```python
from build123d import *

# Parameters (mm, degrees)
SCHIZZO1_R                   = 4
SCHIZZO1_R_2                 = 10.5
SCHIZZO1_R_3                 = 3
ESTRUSIONE_ESTRUSIONE2_DEPTH = 10
SCHIZZO2_R                   = 2
TAGLIO_ESTRUSIONE1_DEPTH     = 15


with BuildPart() as part:
    # Schizzo1 → Estrusione-Estrusione2 (new body)
    with BuildSketch(Plane.XY):
        with BuildLine():
            Line((20, 0), (87.022408988, 0))
            ThreePointArc((87.022408988, 0), (97.768401155, 3.132171084), (105.148564729, 11.547634765))
            Line((105.148564729, 11.547634765), (242.445343973, 305.981528018))
            ThreePointArc((242.445343973, 305.981528018), (243.845108375, 310.105100974), (244.319188233, 314.433893253))
            Line((244.319188233, 314.433893253), (244.319188233, 380))
            ThreePointArc((244.319188233, 380), (238.461323856, 394.142135624), (224.319188233, 400))
            Line((224.319188233, 400), (166.622932407, 400))
            ThreePointArc((166.622932407, 400), (155.87694024, 396.867828916), (148.496776667, 388.452365235))
            Line((148.496776667, 388.452365235), (1.873844259, 74.018471982))
            ThreePointArc((1.873844259, 74.018471982), (0.474079858, 69.894899026), (0, 65.566106747))
            Line((0, 65.566106747), (0, 20))
            ThreePointArc((0, 20), (5.857864376, 5.857864376), (20, 0))
        make_face()
        with Locations((39.213445393, 53)):
            Circle(SCHIZZO1_R, mode=Mode.SUBTRACT)
        with Locations(Location((65.213445393, 53, 0), (0, 0, 180))):
            Circle(SCHIZZO1_R, mode=Mode.SUBTRACT)
        with Locations((65.213445393, 27)):
            Circle(SCHIZZO1_R, mode=Mode.SUBTRACT)
        with Locations(Location((39.213445393, 27, 0), (0, 0, 180))):
            Circle(SCHIZZO1_R, mode=Mode.SUBTRACT)
        with Locations((199.319188233, 355.469283566)):
            Circle(SCHIZZO1_R_2, mode=Mode.SUBTRACT)
        with Locations((183.819188233, 383.469283566)):
            Circle(SCHIZZO1_R_3, mode=Mode.SUBTRACT)
        with Locations((214.819188233, 383.469283566)):
            Circle(SCHIZZO1_R_3, mode=Mode.SUBTRACT)
        with Locations((220.532391668, 376.682487002)):
            Circle(SCHIZZO1_R_3, mode=Mode.SUBTRACT)
        with Locations((220.532391668, 334.256080131)):
            Circle(SCHIZZO1_R_3, mode=Mode.SUBTRACT)
        with Locations((214.819188233, 327.469283566)):
            Circle(SCHIZZO1_R_3, mode=Mode.SUBTRACT)
        with Locations((183.819188233, 327.469283566)):
            Circle(SCHIZZO1_R_3, mode=Mode.SUBTRACT)
        with Locations((178.105984797, 334.256080131)):
            Circle(SCHIZZO1_R_3, mode=Mode.SUBTRACT)
        with Locations((178.105984797, 376.682487002)):
            Circle(SCHIZZO1_R_3, mode=Mode.SUBTRACT)
    extrude(amount=-ESTRUSIONE_ESTRUSIONE2_DEPTH)

    # Schizzo2 → Taglio-Estrusione1 (cut)
    with BuildSketch(Plane.XZ):
        with Locations((53.511204494, -5)):
            Circle(SCHIZZO2_R)
        with Locations((81.011204494, -5)):
            Circle(SCHIZZO2_R)
        with Locations(Location((26.011204494, -5, 0), (0, 0, 180))):
            Circle(SCHIZZO2_R)
    extrude(amount=-TAGLIO_ESTRUSIONE1_DEPTH, mode=Mode.SUBTRACT)


solid = part.part
```
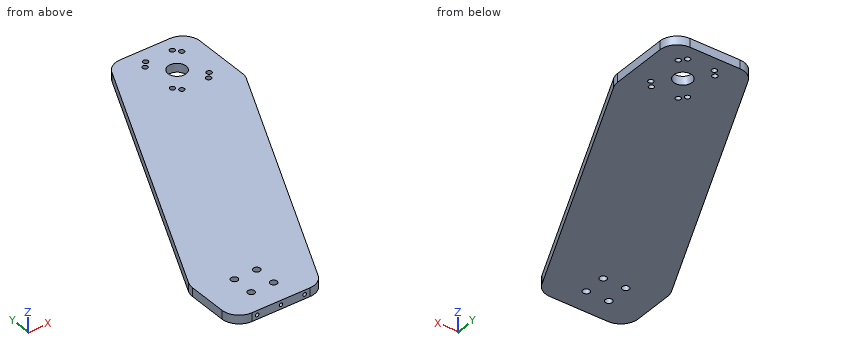
Geometry: final body of the model. Coordinates: model frame, mm. Coordinates: 2 decimals unless noted, no trailing zeros. Order: outer loops, then holes, each group sorted by start corner. A loop starts at its lowest first (then second) coordinate and runs counter-clockwise, first axis right, second up. Notation, with made-up numbers: (28.5, 85.25) - (39.5, 85.25) arc R31 ccw to (39.5, 119.25) - close; hole circle Ø3 at (11, 45.25). An arc over 180 degrees is marked (long way). Write each question's results on one line, items separated by ' | '.
(1) First-contact query: pin 1 Ø4 at (x, z) = (102.5, -8) entering from -Y; pin 2 Ø2.5 at (x, z) = (81.01, -5) entering from +Y; pin 3 Ø5 at (y, z) = (137.5, -1.5) entering from +X. Flat tips, straight axial feed; report the tip coordinate or a pass-through.
Values found:
pin 1: stops at y = 5.22 | pin 2: stops at y = 246.41 | pin 3: stops at x = 165.05
(2) Section query A-A, the plane y = 53. Return the cut outline in (x, z).
Values found:
outline: (0, -10) - (35.21, -10) - (35.21, 0) - (0, 0) - close; (43.21, -10) - (61.21, -10) - (61.21, 0) - (43.21, 0) - close; (69.21, -10) - (124.48, -10) - (124.48, 0) - (69.21, 0) - close
(3) Section query D-D, the plane y = 183. Return the cut outline in (x, z).
Values found:
outline: (52.69, -10) - (185.1, -10) - (185.1, 0) - (52.69, 0) - close
(4) Line query: line 1 (X direction, y = 55.5, z = -3.75); line 2 (Y direction, x = 186, z = -8.25); line 3 (X direction, y = 52, z = -4.75). Output: solid intervals per line, ascending. Write a range as [from, to].
Values found:
line 1: x = [0, 36.09], [42.34, 62.09], [68.34, 125.64] | line 2: y = [184.93, 325.41], [329.53, 381.41], [385.53, 400] | line 3: x = [0, 35.34], [43.09, 61.34], [69.09, 124.01]
(5) Section query C-C, the plane x = 47.5. Return the cut outline in (y, z), plus the area to 3 significant figures.
Values found:
outline: (0, -10) - (171.86, -10) - (171.86, 0) - (0, 0) - close | area: 1,720 mm²
(6) Section query B-B, the plane z = -5. Count the separate pieces of the cut face and the enclosed holes in it, plus the area to 3 significant figures.
Values found:
separate pieces: 1 | enclosed holes: 13 | area: 48,700 mm²
